For this review, take the finished solid that the model builds, in its own axes (mm). A direction names the side the tool comes from. Coordinates: 2 decimals unless noted, no trailing zeros. Loops run counter-clockwise (first coordinate to the right, second up) from the corner with the lowest first, then second, coordinate; pieces in that order, holes last. Notation, with made-up numbers: M 66,33.5 L 112,33.5 A31 ccw 112,58.5 Z; hole C 67.25,72 d6. An arc over 180 degrees is marked long. Answer as a JSON object with one key per item and string values. Group by question number.
Item 1: Add section A-A (x = 0). State the section outline as (y, z) points.
Item 2: Wall thickness on L1, parallel to Y at x = 0, z = -2.5; L2, parallel to Y at x = 0, z = 0.55; L3, parallel to Z at x = -41, y = -12.5: over which ranges is each line inside the solid? List them lowest first. Write a range as from..to.
Item 3: Mouldability with a two-part tool opening along X and no side actions: class faces 1 (the face through (-50, 59, -3)), 2 (the face through (-47.265, 61.034, -1.521)), 3 (the face through (72.975, -0.847, 0.986)), 4 (the face through (-47.076, 55.767, -1.521)) as +X half, -X half, draft (parallel to the pull), parting line (faces both ways), or undercut.
Item 4: Insertion check: pin 1 (3 mm diameter, centred on x = -48.5, z = 0, fed in from -Y); pin 2 (6 mm diameter, centred on x = 7, y = -8, fed in from +Z); pin 3 (1 mm diameter, centred on y = 63, z = -2, fed in from -X). Each pin has a flat end and moves straight along its axis. Give the tip position at first contact, or say it passes through.
Item 5: Add section B-B (y = -45). State the section outline as (x, z) points, then the cut area to 3 significant figures.
Item 6: Add section D-D (y = -13). State the section outline as (x, z) points, then the cut area to 3 significant figures.
Item 7: Tool access review of faces 5 (the face through (13, -1, 0)), 6 (the face through (52.17, 56.9, 0.99)), 7 (the face through (47.34, -61.13, -1.52)), 8 (the face through (50, -59, -3)), 9 (the face through (-14.921, 67.193, -1.479)): name each direction out of +Z, -Z, +X, -X, +Y, -Y from which nothing blocks a thin tool from reaching the whole face with its end or side.
Item 8: Add section C-C (x = -63.5). State the section outline as (y, z) points.
from build123d import *
from build123d.topology import SkipClean

# Parameters (mm, degrees)
CSK_FOR_6_FLAT_HEAD_MACHINE_SCREW_100_D           = 3.7973
CSK_FOR_6_FLAT_HEAD_MACHINE_SCREW_100_CSINK_D     = 7.0866
CSK_FOR_6_FLAT_HEAD_MACHINE_SCREW_100_CSINK_ANGLE = 100
CUT_EXTRUDE1_DEPTH                                = 10
CUT_EXTRUDE2_DEPTH                                = 116.409192875
CUT_EXTRUDE2_DEPTH_BACK                           = 116.409192875
BOSS_EXTRUDE1_START                               = -5
BOSS_EXTRUDE1_DEPTH                               = 5
CUT_EXTRUDE3_DEPTH                                = 10


with BuildPart() as part:
    # Sketch1 → Revolve1 (revolve)
    with BuildSketch(Plane(origin=(0, 0, 0), x_dir=(1, 0, 0), z_dir=(0, 1, 0)), mode=Mode.PRIVATE) as revolve1_sk:
        Polygon((-68.83, 3), (-68.83, 0), (-81.53, 0), (-81.53, -2), (-68.83, -2), (-60.848940548, -2), (-60.848940548, 0), (0, 0), (0, 3), align=None)
    revolve(revolve1_sk.sketch.rotate(Axis((0, 0, 0), (0, 0, -1)), 180), axis=Axis((0, 0, 0), (0, 0, -1)))

    # CSK for #6 Flat Head Machine Screw (100)1 (through all)
    with Locations(Plane(origin=(0, 0.307599269, 0), x_dir=(1, 0, 0), z_dir=(0, 0, 1))):
        with Locations((0, 0)):
            CounterSinkHole(CSK_FOR_6_FLAT_HEAD_MACHINE_SCREW_100_D / 2, CSK_FOR_6_FLAT_HEAD_MACHINE_SCREW_100_CSINK_D / 2, counter_sink_angle=CSK_FOR_6_FLAT_HEAD_MACHINE_SCREW_100_CSINK_ANGLE)

    # Sketch5 → Cut-Extrude1 (cut)
    with BuildSketch(Plane(origin=(0, 0, 0), x_dir=(-1, 0, 0), z_dir=(0, 0, -1))):
        with BuildLine():
            Line((-49.321326643, 53.791143678), (-57.904237692, 63.151893537))
            ThreePointArc((-57.904237692, 63.151893537), (-85.68, 0), (-57.904237692, -63.151893537))
            Line((-57.904237692, -63.151893537), (-49.321326643, -53.791143678))
            ThreePointArc((-49.321326643, -53.791143678), (-72.98, 0), (-49.321326643, 53.791143678))
        make_face()
    extrude(amount=-CUT_EXTRUDE1_DEPTH, mode=Mode.SUBTRACT)

    # Sketch6 → Cut-Extrude2 (cut, two sides: drawn at the far end of the back side and taken through both)
    with BuildSketch(Plane.XY.offset(2).offset(-CUT_EXTRUDE2_DEPTH_BACK)):
        with BuildLine():
            Line((-54.761675773, 59.724532368), (-49.321326643, 53.791143678))
            ThreePointArc((-49.321326643, 53.791143678), (-72.98, 0), (-49.321326643, -53.791143678))
            Line((-49.321326643, -53.791143678), (-54.761675773, -59.724532368))
            ThreePointArc((-54.761675773, -59.724532368), (-81.03, 0), (-54.761675773, 59.724532368))
        make_face()
    extrude(amount=CUT_EXTRUDE2_DEPTH + CUT_EXTRUDE2_DEPTH_BACK, mode=Mode.SUBTRACT)

    # Sketch7 → Boss-Extrude1 (add)
    with SkipClean():  # the faces are left unmerged after this step: merging them gives an invalid solid
        with BuildSketch(Plane.XY.offset(2).offset(BOSS_EXTRUDE1_START)):
            with BuildLine():
                Line((49.321326643, -53.791143678), (55.099585656, -60.093065827))
                ThreePointArc((55.099585656, -60.093065827), (52.554806839, -62.330836495), (49.919235, -64.460925195))
                Line((49.919235, -64.460925195), (44.684236113, -57.700948372))
                ThreePointArc((44.684236113, -57.700948372), (47.043417185, -55.794240738), (49.321326643, -53.791143678))
            make_face()
            with BuildLine():
                Line((-44.684236113, 57.700948372), (-49.919235, 64.460925195))
                ThreePointArc((-49.919235, 64.460925195), (-52.554806839, 62.330836495), (-55.099585656, 60.093065827))
                Line((-55.099585656, 60.093065827), (-49.321326643, 53.791143678))
                ThreePointArc((-49.321326643, 53.791143678), (-47.043417185, 55.794240738), (-44.684236113, 57.700948372))
            make_face()
        extrude(amount=BOSS_EXTRUDE1_DEPTH)

    # Sketch9 → Cut-Extrude3 (cut)
    with BuildSketch(Plane.XY.offset(2)):
        with BuildLine():
            Line((-54.761675773, 59.724532368), (-55.099585656, 60.093065827))
            ThreePointArc((-55.099585656, 60.093065827), (-81.53, 0), (-55.099585656, -60.093065827))
            Line((-55.099585656, -60.093065827), (-54.761675773, -59.724532368))
            ThreePointArc((-54.761675773, -59.724532368), (-81.03, 0), (-54.761675773, 59.724532368))
        make_face()
    extrude(amount=-CUT_EXTRUDE3_DEPTH, mode=Mode.SUBTRACT)


solid = part.part
From the geometry:
{
 "1": {"outline": "M -81.53,0 L -68.83,0 L -68.83,-3 L -1.59,-3 L -1.59,-1.38 L -3.24,0 L -60.85,0 L -60.85,2 L -81.53,2 Z; M 2.21,-3 L 68.83,-3 L 68.83,0 L 81.53,0 L 81.53,2 L 60.85,2 L 60.85,0 L 3.85,0 L 2.21,-1.38 Z"},
 "2": {"L1": "y = -68.83..-1.59, 2.21..68.83", "L2": "y = -81.53..-60.85, 60.85..81.53", "L3": "z = -3..0"},
 "3": {"face 1": "draft", "face 2": "undercut", "face 3": "+X half", "face 4": "undercut"},
 "4": {"pin 1": "stops at y = -66.62", "pin 2": "stops at z = 0", "pin 3": "stops at x = -52.35"},
 "5": {"outline": "M -57.46,0 L -52.08,0 L -52.08,-3 L 52.08,-3 L 52.08,0 L 57.46,0 L 57.46,2 L 40.96,2 L 40.96,0 L -40.96,0 L -40.96,2 L -57.46,2 Z", "area": "378 mm²"},
 "6": {"outline": "M -71.81,0 L -67.59,0 L -67.59,-3 L 67.59,-3 L 67.59,0 L 71.81,0 L 71.81,2 L 59.44,2 L 59.44,0 L -59.44,0 L -59.44,2 L -71.81,2 Z", "area": "455 mm²"},
 "7": {"face 5": "+Z", "face 6": "+Z, -Z, +X", "face 7": "-Z, -Y", "face 8": "-Z, +X, -X, +Y, -Y", "face 9": "-Z"},
 "8": {"outline": "M -35.97,0 L -26.56,0 L -26.56,-3 L 26.56,-3 L 26.56,0 L 35.97,0 L 35.97,2 L -35.97,2 Z"}
}
